```python
from build123d import *

# Parameters (mm, degrees)
BOSS_EXTRUDE1_DEPTH = 0.254
FILLET2_R           = 0.254


with BuildPart() as part:
    # Sketch1 → Boss-Extrude1 (new body)
    with BuildSketch(Plane.XY):
        Polygon((-49.105346889, -48.133448144), (-47.200346889, -48.133448144), (-47.200346889, -54.280248144), (-47.797246889, -54.280248144), (-47.797246889, -57.684193827), (-48.031682458, -58.090248144), (-48.27401132, -58.090248144), (-48.508446889, -57.684193827), (-48.508446889, -54.280248144), (-49.105346889, -54.280248144), align=None)
    extrude(amount=BOSS_EXTRUDE1_DEPTH)

    # Fillet2
    fillet2_edges = [part.edges().sort_by_distance(p)[0] for p in [
        (-49.105346889, -48.133448144, 0.127),
        (-47.200346889, -48.133448144, 0.127),
    ]]
    fillet(fillet2_edges, radius=FILLET2_R)


solid = part.part
```
CAD build for the part. Positions are in the model's coordinates, mm. Give positions to 0.01 mm unless a question says otherwise; leave off trailing zeros. Order: outer loops, then holes, each group sorted by start corner. A loop starts at its lowest first (then second) coordinate and runs counter-clockwise, first axis right, second up.
(1) Saw through at B-B, the plane x = -48.65. Give the cut face in (y, z).
(2) Saw through at C-C, the plane y = -54.5. Give the cut face in (x, z), then the cut area to 3 significant figures.
(3) Drill centre lines: L1, parallel to X at y = -56.75, z = 0.2; L2, parallel to Y at x = -48.55, z = 0.15; L3, parallel to Y at x = -48.3, z = 0.1. Where is each one in solid material? Low to high.
(4) Saw through at A-A, the plane z = 0.15. Give the cut face in (x, y), then the cut area to 3 significant figures.
Results found:
1. outline: (-54.28, 0) - (-48.13, 0) - (-48.13, 0.25) - (-54.28, 0.25) - close
2. outline: (-48.51, 0) - (-47.8, 0) - (-47.8, 0.25) - (-48.51, 0.25) - close
2. area: 0.181 mm2
3. L1: x = -48.51 to -47.8
3. L2: y = -54.28 to -48.13
3. L3: y = -58.05 to -48.13
4. outline: (-49.11, -54.28) - (-48.51, -54.28) - (-48.51, -57.68) - (-48.27, -58.09) - (-48.03, -58.09) - (-47.8, -57.68) - (-47.8, -54.28) - (-47.2, -54.28) - (-47.2, -48.39) arc R0.25 ccw to (-47.45, -48.13) - (-48.85, -48.13) arc R0.25 ccw to (-49.11, -48.39) - close
4. area: 14.3 mm2
